Design review of the part shown in the three views and the two pictorial views. Dimensions are in mm from the part's minimum x, y and z. A direction names the side the tool comes from. Round coordinates to 2 decimals unless told otherwise and drop trailing zeros. Loops run counter-clockwise (first coordinate to the right, second up) from the corner with the lowest first, then second, coordinate; pieces in that order, holes last. Notation, with made-up numbers: M 14.5,12 L 71.5,12 A23 cw 71.5,42 Z; hole C 47,77.5 d6. An arc over 180 degrees is marked long. One line per question, with ' | ' between items. Start each with the question number.
1) Mouldability with a two-part tool opening along X and no side actions: class the marked faces 1, 2 and 3 as pulls with the +X half, pulls with the -X half, needs draft (parallel to the pull), parting line crosses it, or undercut.
2) For pin 1 Ø4 at (x, y) = (39, 23) entering from +Z, flat-tipped, find the tip position at first contact; note if it passes through.
3) We need section A-A (z = 39). Give the boundary of the cut face in (x, y).
4) We need section B-B (y = 46). Give the boundary of the cut face in (x, z).
5) For the marked faces 4 and 5, list the 3-axis set-ups (+Z, -Z, +X, -X, +Y, -Y) from which the entire face can be reached by the end or side of a thin tool; tool diameter is ignored.
6) We need section C-C (x = 40). Give the boundary of the cut face in (y, z).
7) We need section D-D (z = 5). Give the boundary of the cut face in (x, y), and give its area (3 significant figures).
8) For probe 1 along Y at (x, z) = (9.5, 2.2); probe 2 along X at (y, z) = (15.5, 31.5); probe 3 along Y at (x, z) = (25, 0.75), list the stretches that pass through material, from the lowest coordinate up. Write a range as from..to.
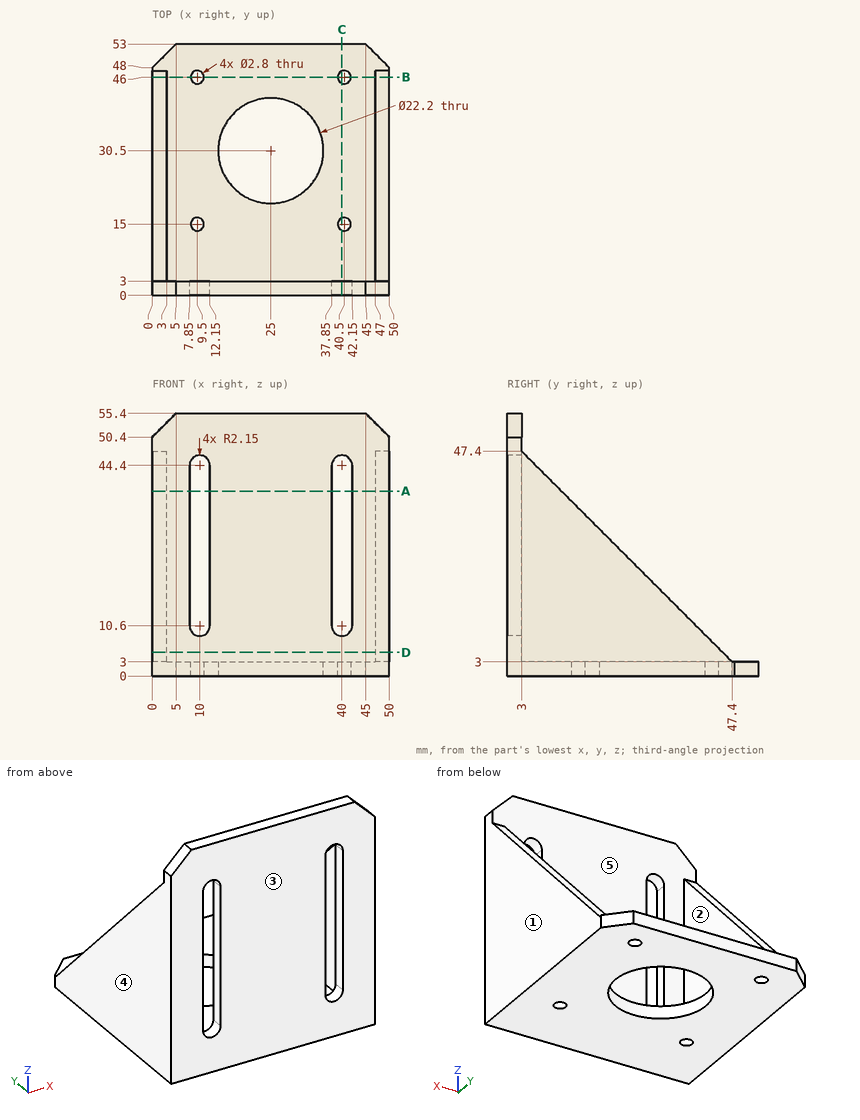
Answers below:
1) face 1: pulls with the +X half | face 2: undercut | face 3: needs draft
2) pin 1: z = 3
3) outline: M 0,0 L 7.85,0 L 7.85,3 L 3,3 L 3,11.4 L 0,11.4 Z; M 12.15,0 L 37.85,0 L 37.85,3 L 12.15,3 Z; M 42.15,0 L 50,0 L 50,11.4 L 47,11.4 L 47,3 L 42.15,3 Z
4) outline: M 0,0 L 8.1,0 L 8.1,3 L 3,3 L 3,4.4 L 0,4.4 Z; M 10.9,0 L 39.1,0 L 39.1,3 L 10.9,3 Z; M 41.9,0 L 50,0 L 50,4.4 L 47,4.4 L 47,3 L 41.9,3 Z
5) face 4: +Z, -Z, -X, +Y, -Y | face 5: +Z, +Y
6) outline: M 0,0 L 13.69,0 L 13.69,3 L 3,3 L 3,8.45 L 0,8.45 Z; M 0,46.55 L 3,46.55 L 3,55.4 L 0,55.4 Z; M 16.31,0 L 44.69,0 L 44.69,3 L 16.31,3 Z; M 47.31,0 L 53,0 L 53,3 L 47.31,3 Z
7) outline: M 0,0 L 50,0 L 50,45.4 L 47,45.4 L 47,3 L 3,3 L 3,45.4 L 0,45.4 Z | area: 404 mm^2
8) probe 1: 0..13.6, 16.4..44.6, 47.4..53 | probe 2: 0..3, 47..50 | probe 3: 0..19.4, 41.6..53
